```python
from build123d import *

# Parameters (mm, degrees)
SZKIC1_W                    = 65.5
SZKIC1_H                    = 114
DODANIE_WYCI_GNI_CIE1_DEPTH = 6
SZKIC2_R                    = 12.5
WYTNIJ_WYCI_GNI_CIE2_DEPTH  = 6
SZKIC4_R                    = 1.55
WYTNIJ_WYCI_GNI_CIE3_DEPTH  = 6
SZKIC5_W                    = 15
SZKIC5_H                    = 10
SZKIC5_W_2                  = 6
SZKIC5_H_2                  = 30
WYTNIJ_WYCI_GNI_CIE4_DEPTH  = 6
WYTNIJ_WYCI_GNI_CIE5_DEPTH  = 6
WYTNIJ_WYCI_GNI_CIE6_DEPTH  = 6
SZKIC8_R                    = 11.5
WYTNIJ_WYCI_GNI_CIE7_DEPTH  = 10


with BuildPart() as part:
    # Szkic1 → Dodanie-wyciągnięcie1 (new body)
    with BuildSketch(Plane.XY):
        with Locations((23.742718173, 26.167032616)):
            Rectangle(SZKIC1_W, SZKIC1_H)
    extrude(amount=DODANIE_WYCI_GNI_CIE1_DEPTH)

    # Szkic2 → Wytnij-wyciągnięcie2 (cut)
    with BuildSketch(Plane.XY.offset(6)):
        with Locations((32.562718173, 4.504913836)):
            Circle(SZKIC2_R)
    extrude(amount=-WYTNIJ_WYCI_GNI_CIE2_DEPTH, mode=Mode.SUBTRACT)

    # Szkic4 → Wytnij-wyciągnięcie3 (cut)
    with BuildSketch(Plane(origin=(0, 0, 0), x_dir=(-1, 0, 0), z_dir=(0, 0, -1))):
        with Locations((-17.062718173, -10.995086164)):
            Circle(SZKIC4_R)
        with Locations((-17.062718173, 20.004913836)):
            Circle(SZKIC4_R)
        with Locations((-48.062718173, 20.004913836)):
            Circle(SZKIC4_R)
        with Locations((-48.062718173, -10.995086164)):
            Circle(SZKIC4_R)
    extrude(amount=-WYTNIJ_WYCI_GNI_CIE3_DEPTH, mode=Mode.SUBTRACT)

    # Szkic5 → Wytnij-wyciągnięcie4 (cut)
    with BuildSketch(Plane.XY.offset(6)):
        Polygon((-9.007281827, 4.167032616), (-9.007281827, -30.832967384), (6.992718173, -30.832967384), (6.992718173, 4.167032616), (-3.007281827, 4.167032616), align=None)
        with Locations((28.492718173, -25.832967384)):
            Rectangle(SZKIC5_W, SZKIC5_H)
        Polygon((56.492718173, 77.167032616), (56.492718173, 83.167032616), (-9.007281827, 83.167032616), (-9.007281827, 64.167032616), (-3.007281827, 64.167032616), (-3.007281827, 77.167032616), align=None)
        with Locations((-6.007281827, 29.167032616)):
            Rectangle(SZKIC5_W_2, SZKIC5_H_2)
    extrude(amount=-WYTNIJ_WYCI_GNI_CIE4_DEPTH, mode=Mode.SUBTRACT)

    # Szkic6 → Wytnij-wyciągnięcie5 (cut)
    with BuildSketch(Plane.XY.offset(6)):
        Polygon((-3.007281827, 31.667032616), (4.492718173, 31.667032616), (4.492718173, 33.042032616), (6.492718173, 33.042032616), (6.492718173, 31.667032616), (6.992718173, 31.667032616), (6.992718173, 28.567032616), (6.492718173, 28.567032616), (6.492718173, 27.192032616), (4.492718173, 27.192032616), (4.492718173, 28.567032616), (-3.007281827, 28.567032616), align=None)
        Polygon((26.892718173, -20.832967384), (29.992718173, -20.832967384), (29.992718173, -12.332967384), (31.367718173, -12.332967384), (31.367718173, -10.332967384), (29.992718173, -10.332967384), (29.992718173, -9.832967384), (26.892718173, -9.832967384), (26.892718173, -10.332967384), (25.517718173, -10.332967384), (25.517718173, -12.332967384), (26.892718173, -12.332967384), align=None)
    extrude(amount=-WYTNIJ_WYCI_GNI_CIE5_DEPTH, mode=Mode.SUBTRACT)

    # Szkic7 → Wytnij-wyciągnięcie6 (cut)
    with BuildSketch(Plane.XY.offset(6)):
        Polygon((56.492718173, 33.717032616), (48.992718173, 33.717032616), (48.992718173, 35.092032616), (46.992718173, 35.092032616), (46.992718173, 33.717032616), (46.492718173, 33.717032616), (46.492718173, 30.617032616), (46.992718173, 30.617032616), (46.992718173, 29.242032616), (48.992718173, 29.242032616), (48.992718173, 30.617032616), (56.492718173, 30.617032616), align=None)
        Polygon((21.942718173, 69.667032616), (20.567718173, 69.667032616), (20.567718173, 67.667032616), (21.942718173, 67.667032616), (21.942718173, 67.167032616), (25.042718173, 67.167032616), (25.042718173, 67.667032616), (26.417718173, 67.667032616), (26.417718173, 69.667032616), (25.042718173, 69.667032616), (25.042718173, 77.167032616), (21.942718173, 77.167032616), align=None)
    extrude(amount=-WYTNIJ_WYCI_GNI_CIE6_DEPTH, mode=Mode.SUBTRACT)

    # Szkic8 → Wytnij-wyciągnięcie7 (cut)
    with BuildSketch(Plane.XY.offset(6)):
        with Locations((32.562718173, 51.504913836)):
            Circle(SZKIC8_R)
    extrude(amount=-WYTNIJ_WYCI_GNI_CIE7_DEPTH, mode=Mode.SUBTRACT)


solid = part.part
```
Geometry: final body of the model. Coordinates: model frame, mm. A direction names the side the tool comes from. Round coordinates to 2 decimals unless told otherwise and drop trailing zeros. Loops run counter-clockwise (first coordinate to the right, second up) from the corner with the lowest first, then second, coordinate; pieces in that order, holes last. Notation, with made-up numbers: (35, 24) -> (63, 24) arc R9 cw to (63, 30) -> close; hole circle Ø11 at (1, 26.5). An arc over 180 degrees is marked (long way). Use one line per item in the form item = value.
Item 1: Cut plane A-A on x = -0.5. Output: boundary loops of the cut face in (y, z).
Evaluation:
outline = (4.17, 0) -> (28.57, 0) -> (28.57, 6) -> (4.17, 6) -> close; (31.67, 0) -> (77.17, 0) -> (77.17, 6) -> (31.67, 6) -> close
Item 2: Cut plane C-C on y = 23. Output: boundary loops of the cut face in (x, z), then the cut area to 3 significant figures.
Evaluation:
outline = (-3.01, 0) -> (56.49, 0) -> (56.49, 6) -> (-3.01, 6) -> close
area = 357 mm2
Item 3: Cut plane B-B on y = 7. Output: boundary loops of the cut face in (x, z), then the cut area to 3 significant figures.
Evaluation:
outline = (-9.01, 0) -> (20.31, 0) -> (20.31, 6) -> (-9.01, 6) -> close; (44.81, 0) -> (56.49, 0) -> (56.49, 6) -> (44.81, 6) -> close
area = 246 mm2
Item 4: Contact query for flat-ended pins moving along their axis: pin 1 Ø1.5 at (x, z) = (22.5, 1) entering from -Y; pin 2 Ø3 at (y, z) = (73.5, 2.5) entering from -X; pin 3 Ø1.8 at (x, z) = (1.5, 2) entering from -Y; pin 4 Ø22.5 at (x, y) = (32.56, 4.5) entering from +Z. Output: stop coordinate, or through.
Evaluation:
pin_1 = -20.83
pin_2 = -3.01
pin_3 = 4.17
pin_4 = through
Item 5: Access query for faces 5 (the flat face through (48, 29.242, 3)), 6 (the flat face through (1, 31.667, 3)), 7 (the flat face through (-6, 64.167, 3)), 8 (the flat face through (29.993, -17, 3)), 9 (the flat face through (46.493, 32, 3)). Directions: +Z, -Z, +X, -X, +Y, -Y. A direction counts if a zero-diameter tool reaches every point of the face in a straight line with its end or side. Return the directions, or none.
Evaluation:
face_5 = +Z, -Z
face_6 = +Z, -Z, -X
face_7 = +Z, -Z, -X, +Y
face_8 = +Z, -Z, -Y
face_9 = +Z, -Z, +X
Item 6: Draft query along Y for faces 1 (the flat face through (26.418, 69, 3)), 2 (the flat face through (24, -20.833, 3)), 3 (the flat face through (25.518, -11, 3)), 4 (the flat face through (23, 67.167, 3)). Return one class per face: released by +Y, released by -Y, zero draft, split by the parting line, or undercut.
Evaluation:
face_1 = undercut
face_2 = released by -Y
face_3 = undercut
face_4 = released by +Y
Item 7: Material intervals for probe 1 along X at (y, z) = (-11, 1.5); probe 2 along X at (y, z) = (51, 0.9); probe 3 along Y at (x, z) = (3.5, 0.8), sorted ascending.
Evaluation:
probe_1 = 6.99 to 15.51, 18.61 to 25.52, 31.37 to 46.51, 49.61 to 56.49
probe_2 = -9.01 to 21.07, 44.05 to 56.49
probe_3 = 4.17 to 28.57, 31.67 to 77.17
Item 8: Cut plane D-D on z = 2.35. Give the number of separate pieces and of enclosed holes in the cut face, then the cut area to 3 significant figures.
Evaluation:
separate_pieces = 1
enclosed_holes = 6
area = 5,020 mm2
